Study the drawing (mm; zero at the part's minimum x, y, z) and answer. A direction names the side the tool comes from. Coordinates: 2 decimals unless noted, no trailing zeros. Loops run counter-clockwise (first coordinate to the right, second up) from the corner with the lowest first, then second, coordinate; pieces in that order, holes last.
Q1. Section C-C (x = 36) is taken. Give the vertices of the cut face in (y, z).
Q2. Straight lines are drawn through the part: line 1 (X direction, y = 1.55, z = 45); line 2 (Z direction, x = 12.5, y = 8.75); line 3 (Z direction, x = 3, y = 11.75). For each, find the intervals that lie inside material, in ascending order.
Q3. Flat-ended cylindrical pins translate along their axes: P1, Ø2.5, axis at y = 13, z = 28, coming from the -X side; P2, Ø0.6, axis at y = 12.5, z = 13, coming from the -X side; P3, Ø1, axis at x = 37.5, y = 10.5, coming from the -Z side. Find the tip coordinate at first contact, or state that the pin passes through.
Q4. Section A-A (z = 19.5) is taken. Give the vertices of the cut face in (x, y).
Q5. Which of the six approach directions +Z, -Z, +X, -X, +Y, -Y give full straight-line access (tool end or side, diameter ignored) to the marked faces 1, 2, 3, 4 and 5?
Q6. The mould has two halves that part along Z. Classify the marked faces 6, 7 and 8: pulls with the +Z half, pulls with the -Z half, needs draft (parallel to the pull), parting line crosses it, or undercut.
Q7. Section B-B (x = 21) is taken. Give the vertices of the cut face in (y, z), then the cut area to 3 significant figures.
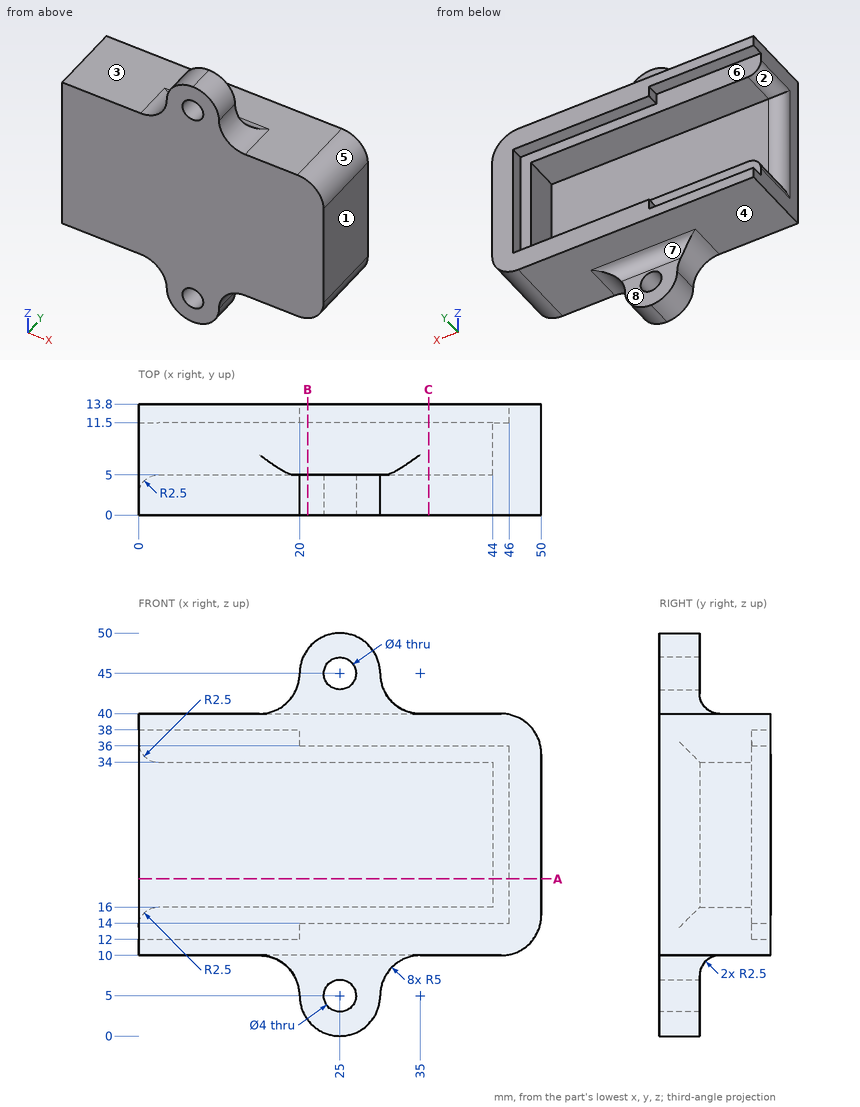
Numbers:
1. outline: (0, 10) - (13.8, 10) - (13.8, 14) - (11.5, 14) - (11.5, 16) - (5, 16) - (5, 34) - (11.5, 34) - (11.5, 36) - (13.8, 36) - (13.8, 40) - (0, 40) - close
2. line 1: x = 20 to 23, 27 to 30
2. line 2: z = 10 to 16, 34 to 40
2. line 3: z = 10 to 12, 38 to 40
3. P1: stops at x = 46
3. P2: stops at x = 20
3. P3: stops at z = 10
4. outline: (0, 0) - (50, 0) - (50, 13.8) - (46, 13.8) - (46, 11.5) - (44, 11.5) - (44, 5) - (2.5, 5) arc R2.5 ccw to (0, 2.5) - close
5. face 1: +Z, -Z, +X, +Y, -Y
5. face 2: -X, +Y
5. face 3: +Z, +Y
5. face 4: -Z, +Y
5. face 5: +Z, +X, +Y, -Y
6. face 6: undercut
6. face 7: pulls with the -Z half
6. face 8: needs draft
7. outline: (0, 2) - (5, 2) - (5, 7.5) arc R2.5 cw to (7.5, 10) - (13.8, 10) - (13.8, 14) - (11.5, 14) - (11.5, 16) - (5, 16) - (5, 34) - (11.5, 34) - (11.5, 36) - (13.8, 36) - (13.8, 40) - (7.5, 40) arc R2.5 cw to (5, 42.5) - (5, 48) - (0, 48) - close
7. area: 329 mm2
